from build123d import *

# Parameters (mm, degrees)
F1_DEPTH = 30
F2_R     = 12.75
F3_DEPTH = 30


with BuildPart() as f1:
    # F0 (on Top) → F1 (new body)
    with BuildSketch(Plane.XY):
        with BuildLine():
            ThreePointArc((28.1024909928, -10.5), (29.5218116804, -5.3350384355), (30, 0))
            ThreePointArc((30, 0), (29.5218116804, 5.3350384355), (28.1024909928, 10.5))
            Line((28.1024909928, 10.5), (28.1024909928, -10.5))
        make_face()
        with BuildLine():
            Line((21.5812418549, 10.5), (28.1024909928, 10.5))
            ThreePointArc((28.1024909928, 10.5), (26.747487876, 13.5857238424), (25.0549396327, 16.5))
            Line((25.0549396327, 16.5), (17.4284250579, 16.5))
            ThreePointArc((17.4284250579, 16.5), (19.7341969222, 13.6587507422), (21.5812418549, 10.5))
        make_face()
        with BuildLine():
            Line((28.1024909928, -10.5), (28.1024909928, 10.5))
            Line((28.1024909928, 10.5), (21.5812418549, 10.5))
            ThreePointArc((21.5812418549, 10.5), (23.3874945699, 5.3874945699), (24, 0))
            ThreePointArc((24, 0), (23.3874945699, -5.3874945699), (21.5812418549, -10.5))
            Line((21.5812418549, -10.5), (28.1024909928, -10.5))
        make_face()
        with BuildLine():
            ThreePointArc((25.0549396327, -16.5), (26.747487876, -13.5857238424), (28.1024909928, -10.5))
            Line((28.1024909928, -10.5), (21.5812418549, -10.5))
            ThreePointArc((21.5812418549, -10.5), (19.7341969222, -13.6587507422), (17.4284250579, -16.5))
            Line((17.4284250579, -16.5), (25.0549396327, -16.5))
        make_face()
        with BuildLine():
            Line((17.4284250579, 16.5), (25.0549396327, 16.5))
            ThreePointArc((25.0549396327, 16.5), (-30, 0), (25.0549396327, -16.5))
            Line((25.0549396327, -16.5), (17.4284250579, -16.5))
            ThreePointArc((17.4284250579, -16.5), (-24, 0), (17.4284250579, 16.5))
        make_face()
        with BuildLine():
            Line((3.1024909928, 10.5), (21.5812418549, 10.5))
            ThreePointArc((21.5812418549, 10.5), (19.7341969222, 13.6587507422), (17.4284250579, 16.5))
            Line((17.4284250579, 16.5), (-2.8975090072, 16.5))
            Line((-2.8975090072, 16.5), (-2.8975090072, -16.5))
            Line((-2.8975090072, -16.5), (17.4284250579, -16.5))
            ThreePointArc((17.4284250579, -16.5), (19.7341969222, -13.6587507422), (21.5812418549, -10.5))
            Line((21.5812418549, -10.5), (3.1024909928, -10.5))
            Line((3.1024909928, -10.5), (3.1024909928, 10.5))
        make_face()
    extrude(amount=F1_DEPTH)

    # F2 (on face) → F3 (cut)
    with BuildSketch(Plane.YZ.offset(3.1024909928)):
        with Locations((0, 15)):
            Circle(F2_R)
    extrude(amount=F3_DEPTH, mode=Mode.SUBTRACT)


solid = f1.part
For this review, take the finished solid that the model builds, in its own axes (mm). A direction names the side the tool comes from. Round coordinates to 2 decimals unless told otherwise and drop trailing zeros. Loops run counter-clockwise (first coordinate to the right, second up) from the corner with the lowest first, then second, coordinate; pieces in that order, holes last. Notation, with made-up numbers: (59, 77.5) - (111, 77.5) arc R17 cw to (111, 97.5) - close; hole circle Ø3 at (-36, 38). An arc over 180 degrees is marked (long way). One line per question, with ' | ' between items.
Q1. Take a section at B-B (y = -14). Give the boundary of the cut face in (x, z).
Taken from the geometry:
outline: (-26.53, 0) - (-19.49, 0) - (-19.49, 30) - (-26.53, 30) - close; (-2.9, 0) - (26.53, 0) - (26.53, 30) - (-2.9, 30) - close
Q2. For line 1 along Y through (x, z) = (0, 10); line 2 along X through (y, z) = (0, 19.5); line 3 along Y through (x, z) = (14.5, 27), list the stretches that pass through material, from the lowest coordinate up. Write a range as [from, to].
Taken from the geometry:
line 1: y = [-30, -24], [-16.5, 16.5], [24, 30] | line 2: x = [-30, -24], [-2.9, 3.1] | line 3: y = [-26.26, -19.12], [-16.5, -10.5], [10.5, 16.5], [19.12, 26.26]
Q3. Take a section at A-A (x = 0). Give the boundary of the cut face in (y, z), and give its area (3 significant figures).
Taken from the geometry:
outline: (-30, 0) - (-24, 0) - (-24, 30) - (-30, 30) - close; (-16.5, 0) - (16.5, 0) - (16.5, 30) - (-16.5, 30) - close; (24, 0) - (30, 0) - (30, 30) - (24, 30) - close | area: 1,350 mm²
Q4. The part is to be moulded in two halves that separate along Y. For faces 1 (the cylindrical face through (19.35, 12.16, 18.83)), 2 (the flat face through (0, 0, 30)), say which applies: released by +Y, released by -Y, zero draft, split by the parting line, or undercut.
Taken from the geometry:
face 1: undercut | face 2: zero draft
Q5. Take a section at D-D (z = 25.5). Give the boundary of the cut face in (x, y).
Taken from the geometry:
outline: (3.1, -10.5) - (3.1, 10.5) - (21.58, 10.5) arc R24 cw to (22.88, 7.23) - (29.12, 7.23) arc R30 ccw (long way) to (29.12, -7.23) - (22.88, -7.23) arc R24 cw to (21.58, -10.5) - close; hole (-2.9, -16.5) - (-2.9, 16.5) - (17.43, 16.5) arc R24 ccw (long way) to (17.43, -16.5) - close
Q6. Tool access review of faces 3 (the flat face through (0, 0, 0)), 4 (the flat face through (12, 10.5, 26)): name each direction out of +Z, -Z, +X, -X, +Y, -Y from which nothing blocks a thin tool from reaching the whole face with its end or side.
Taken from the geometry:
face 3: -Z, +X, -X, +Y, -Y | face 4: +Z, -Z
Q7. For pin 1 (9 mm diameter, centred on y = 2, z = 14, fed in from -X); pin 2 (16.5 mm diameter, centred on x = 5, z = 12, fed in from -Y); pin 3 (2 mm diameter, centred on x = -14, z = 15, fed in from +Y); pin 4 (5 mm diameter, centred on x = -2, z = 11.5, fed in from +Y), all flat-tipped, find the tip position at first contact; note any pin that passes through.
Taken from the geometry:
pin 1: stops at x = -30 | pin 2: stops at y = -30 | pin 3: stops at y = 27.04 | pin 4: stops at y = 30
Q8. Take a section at C-C (x = 8). Give the boundary of the cut face in (y, z).
Taken from the geometry:
outline: (-28.91, 0) - (-22.63, 0) - (-22.63, 30) - (-28.91, 30) - close; (-16.5, 0) - (-10.5, 0) - (-10.5, 7.77) arc R12.75 cw to (-10.5, 22.23) - (-10.5, 30) - (-16.5, 30) - close; (10.5, 0) - (16.5, 0) - (16.5, 30) - (10.5, 30) - (10.5, 22.23) arc R12.75 cw to (10.5, 7.77) - close; (22.63, 0) - (28.91, 0) - (28.91, 30) - (22.63, 30) - close
